from build123d import *

# Parameters (mm, degrees)
FILLET1_R = 0.508


with BuildPart() as part:
    # Sketch4 → Revolve4 (revolve)
    with BuildSketch(Plane(origin=(0, 0, 0), x_dir=(0, 0, -1), z_dir=(1, 0, 0)), mode=Mode.PRIVATE) as revolve4_sk:
        with BuildLine():
            Line((-3.307050371, 0), (25.4, 0))
            Line((25.4, 0), (25.4, 2.54))
            Line((25.4, 2.54), (0, 2.54))
            Line((0, 2.54), (0, 3.81))
            ThreePointArc((0, 3.81), (-2.694076836, 2.694076836), (-3.81, 0))
            Line((-3.81, 0), (-3.307050371, 0))
        make_face()
    revolve(revolve4_sk.sketch.rotate(Axis((0, 0, 3.307050371), (0, 0, -1)), 90), axis=Axis((0, 0, 3.307050371), (0, 0, -1)))

    # Fillet1
    fillet1_edges = [part.edges().sort_by_distance(p)[0] for p in [
        (-3.81, 0, 0),
        (-2.54, 0, 0),
        (-2.54, 0, -25.4),
    ]]
    fillet(fillet1_edges, radius=FILLET1_R)


solid = part.part
Check sheet for the modelled part. Datum: model origin and axes. Units: mm. A direction names the side the tool comes from. Round coordinates to 2 decimals unless told otherwise and drop trailing zeros. Loops run counter-clockwise (first coordinate to the right, second up) from the corner with the lowest first, then second, coordinate; pieces in that order, holes last. Notation, with made-up numbers: (55.5, 41.25) -> (96.5, 41.25) arc R27 ccw to (96.5, 79.25) -> close; hole circle Ø5 at (-19.75, 68). An arc over 180 degrees is marked (long way). Put each result on its own line as item: value. Start each with the question number.
1. Section check A-A (z = -11.5). Enter the section's corners in (x, y), plus the area to 3 significant figures.
2. Gauge pin test, flat ends, axial feed: pin 1 (2 mm diameter, centred on x = 0.5, y = -1.5, fed in from +Z); pin 2 (1.5 mm diameter, centred on x = -2.5, z = -18, fed in from -Y). Record the tip position at first contact, or that the pin passes through.
3. Access from +Z, -Z, +X, -X, +Y, -Y to the whole of each face (thin tool, end or side, straight path). Record for faces 1 (the face through (0, 0, -25.4)), 2 (the face through (-0.33, -2.52, -12.53)).
4. Scan lines: probe 1 along Y at (x, z) = (-2.25, -0.75); probe 2 along Z at (x, y) = (0.75, -2). Record each from-to range of solid material in increasing order.
Findings:
1. outline: circle Ø5.08 at (0, 0)
1. area: 20.3 mm^2
2. pin 1: stops at z = 3.77
2. pin 2: stops at y = -1.84
3. face 1: -Z, +X, -X, +Y, -Y
3. face 2: -Z
4. probe 1: y = -1.18 to 1.18
4. probe 2: z = -25.39 to 3.15
